Build history of the part. All positions in model axes, mm. A direction names the side the tool comes from. Round coordinates to 2 decimals unless told otherwise and drop trailing zeros. Write each loop counter-clockwise with the first axis right and the second up, starting at its lowest first coordinate (ties: lowest second). Pieces come first, ordered by that corner, then holes. Notation, with made-up numbers: M -6,35.25 L 28,35.25 A19 ccw 28,46.25 Z; hole C 12,80.5 d11. An arc over 180 degrees is marked long. Use a Markdown table: item, result.
from build123d import *

# Parameters (mm, degrees)
BOX001_W          = 5
BOX001_H          = 3
BOX001_DEPTH      = 10
BOX002_W          = 5
BOX002_H          = 3
BOX002_DEPTH      = 10
BOX003_W          = 5
BOX003_H          = 3
BOX003_DEPTH      = 10
CYLINDER_R        = 3.25
CYLINDER_DEPTH    = 10
CYLINDER002_R     = 1
CYLINDER002_DEPTH = 20
CYLINDER001_R     = 1
CYLINDER001_DEPTH = 20
CYLINDER004_R     = 1
CYLINDER004_DEPTH = 20
CYLINDER003_R     = 1
CYLINDER003_DEPTH = 20
CYLINDER006_R     = 1
CYLINDER006_DEPTH = 20
CYLINDER005_R     = 1
CYLINDER005_DEPTH = 20
CYLINDER008_R     = 1
CYLINDER008_DEPTH = 20
CYLINDER007_R     = 1
CYLINDER007_DEPTH = 20
BOX_W             = 29
BOX_H             = 8
BOX_DEPTH         = 11
FILLET_R          = 2


with BuildPart() as cube001:
    # Box001 → Box001 (new body)
    with BuildSketch(Plane(origin=(2, 1.5, 9), x_dir=(1, 0, 0), z_dir=(0, 0, 1))):
        with Locations((2.5, 1.5)):
            Rectangle(BOX001_W, BOX001_H)
    extrude(amount=BOX001_DEPTH)


with BuildPart() as cube002:
    # Box002 → Box002 (new body)
    with BuildSketch(Plane(origin=(8.35, 1.5, 9), x_dir=(1, 0, 0), z_dir=(0, 0, 1))):
        with Locations((2.5, 1.5)):
            Rectangle(BOX002_W, BOX002_H)
    extrude(amount=BOX002_DEPTH)


with BuildPart() as cube003:
    # Box003 → Box003 (new body)
    with BuildSketch(Plane(origin=(22.32, 1.5, 9), x_dir=(1, 0, 0), z_dir=(0, 0, 1))):
        with Locations((2.5, 1.5)):
            Rectangle(BOX003_W, BOX003_H)
    extrude(amount=BOX003_DEPTH)


with BuildPart() as cylinder:
    # Cylinder → Cylinder (new body)
    with BuildSketch(Plane(origin=(17, 3, 9), x_dir=(1, 0, 0), z_dir=(0, 0, 1))):
        Circle(CYLINDER_R)
    extrude(amount=CYLINDER_DEPTH)


with BuildPart() as cylinder002:
    # Cylinder002 → Cylinder002 (new body)
    with BuildSketch(Plane(origin=(5.75, 3, 0), x_dir=(1, 0, 0), z_dir=(0, 0, 1))):
        Circle(CYLINDER002_R)
    extrude(amount=CYLINDER002_DEPTH)


with BuildPart() as fusion:
    # Cylinder001 → Cylinder001 (new body)
    with BuildSketch(Plane(origin=(3.25, 3, 0), x_dir=(1, 0, 0), z_dir=(0, 0, 1))):
        Circle(CYLINDER001_R)
    extrude(amount=CYLINDER001_DEPTH)

    # Fusion: union Cylinder002
    add(cylinder002.part)


with BuildPart() as cylinder004:
    # Cylinder004 → Cylinder004 (new body)
    with BuildSketch(Plane(origin=(5.75, 3, 0), x_dir=(1, 0, 0), z_dir=(0, 0, 1))):
        Circle(CYLINDER004_R)
    extrude(amount=CYLINDER004_DEPTH)


with BuildPart() as fusion001:
    # Cylinder003 → Cylinder003 (new body)
    with BuildSketch(Plane(origin=(3.25, 3, 0), x_dir=(1, 0, 0), z_dir=(0, 0, 1))):
        Circle(CYLINDER003_R)
    extrude(amount=CYLINDER003_DEPTH)

    # Fusion001: union Cylinder004
    add(cylinder004.part)


with BuildPart() as fusion001_1:
    # Fusion001 placement: moved
    add(fusion001.part.moved(Location((6.25, 0, 0))))


with BuildPart() as cylinder006:
    # Cylinder006 → Cylinder006 (new body)
    with BuildSketch(Plane(origin=(5.75, 3, 0), x_dir=(1, 0, 0), z_dir=(0, 0, 1))):
        Circle(CYLINDER006_R)
    extrude(amount=CYLINDER006_DEPTH)


with BuildPart() as fusion002:
    # Cylinder005 → Cylinder005 (new body)
    with BuildSketch(Plane(origin=(3.25, 3, 0), x_dir=(1, 0, 0), z_dir=(0, 0, 1))):
        Circle(CYLINDER005_R)
    extrude(amount=CYLINDER005_DEPTH)

    # Fusion002: union Cylinder006
    add(cylinder006.part)


with BuildPart() as fusion002_1:
    # Fusion002 placement: moved
    add(fusion002.part.moved(Location((20.25, 0, 0))))


with BuildPart() as cylinder008:
    # Cylinder008 → Cylinder008 (new body)
    with BuildSketch(Plane(origin=(5.75, 3, 0), x_dir=(1, 0, 0), z_dir=(0, 0, 1))):
        Circle(CYLINDER008_R)
    extrude(amount=CYLINDER008_DEPTH)


with BuildPart() as fusion004:
    # Cylinder007 → Cylinder007 (new body)
    with BuildSketch(Plane(origin=(3.25, 3, 0), x_dir=(1, 0, 0), z_dir=(0, 0, 1))):
        Circle(CYLINDER007_R)
    extrude(amount=CYLINDER007_DEPTH)

    # Fusion003: union Cylinder008
    add(cylinder008.part)


with BuildPart() as fusion004_1:
    # Fusion003 placement: moved
    add(fusion004.part.moved(Location((12.5, 0, 0))))

    # Fusion004: union Cube001, Cube002, Cube003, Cylinder, Fusion, Fusion001, Fusion002
    add(cube001.part)
    add(cube002.part)
    add(cube003.part)
    add(cylinder.part)
    add(fusion.part)
    add(fusion001_1.part)
    add(fusion002_1.part)


with BuildPart() as standoff:
    # Box → Box (new body)
    with BuildSketch(Plane(origin=(0, -1, 0), x_dir=(1, 0, 0), z_dir=(0, 0, 1))):
        with Locations((14.5, 4)):
            Rectangle(BOX_W, BOX_H)
    extrude(amount=BOX_DEPTH)

    # Fillet
    fillet_edges = [standoff.edges().sort_by_distance(p)[0] for p in [
        (0, -1, 5.5),
        (0, 3, 11),
        (0, 7, 5.5),
        (29, -1, 5.5),
        (29, 3, 11),
        (29, 7, 5.5),
        (14.5, -1, 11),
        (14.5, 7, 11),
    ]]
    fillet(fillet_edges, radius=FILLET_R)

    # Cut: cut Fusion004
    add(fusion004_1.part, mode=Mode.SUBTRACT)


solid = standoff.part
Q1. Cut at B-B on x = 26. Give the cut face in (y, z).
Response values:
| item | result |
|---|---|
| outline | M -1,0 L 2,0 L 2,9 L 1.5,9 L 1.5,11 L 1,11 A2 ccw -1,9 Z; M 4,0 L 7,0 L 7,9 A2 ccw 5,11 L 4.5,11 L 4.5,9 L 4,9 Z |
Q2. Drop flat-ended pins along their axis: P1, Ø1.6, axis at x = 23.5, y = 3, coming from the -Z side (3 decimals); P2, Ø0.9, axis at x = 10, y = 2.5, coming from the +Z side; P3, Ø1.6, axis at x = 25.5, z = 10.5, coming from the -Y side; P4, Ø1.6, axis at y = 2.5, z = 10, coming from the -X side. Give the stop position or say it passes through.
Response values:
| item | result |
|---|---|
| P1 | passes through |
| P2 | stops at z = 9 |
| P3 | stops at y = -0.87 |
| P4 | stops at x = 0.01 |
Q3. Cut at D-D on y = 0.25. Give the cut face in (x, z).
Response values:
| item | result |
|---|---|
| outline | M 0.15,0 L 28.85,0 L 28.85,9 A1.85 ccw 27,10.85 L 18.73,10.85 L 18.73,9 L 15.27,9 L 15.27,10.85 L 2,10.85 A1.85 ccw 0.15,9 Z |
Q4. Drill centre lines: L1, parallel to Y at x = 9.5, z = 5; L2, parallel to Z at x = 18, y = 4.5; L3, parallel to X at y = 3, z = 9.85. Where is each one in solid material? Low to high.
Response values:
| item | result |
|---|---|
| L1 | y = -1 to 2, 4 to 7 |
| L2 | z = 0 to 9 |
| L3 | x = 0.19 to 2, 7 to 8.35, 13.35 to 13.75, 20.25 to 22.32, 27.32 to 28.81 |
Q5. Two-plate mould, pull along X, no slides. Class faces 3 (the flat face through (2, 3, 10)), 4 (the flat face through (22, 3, 11)), 5 (the cylindrical face through (0.57, 6.4, 4.56)): +X half, -X half, draft (parallel to the pull), parting line (faces both ways), or undercut.
Response values:
| item | result |
|---|---|
| face 3 | undercut |
| face 4 | draft |
| face 5 | -X half |
Q6. Cut at A-A on z = 8. Count the separate pieces of the cut face and the enclosed holes in it, and give its area (3 significant figures).
Response values:
| item | result |
|---|---|
| separate pieces | 1 |
| enclosed holes | 8 |
| area | 203 mm2 |
Q7. Which spindle directions (+Z, -Z, +X, -X, +Y, -Y) get a long thin tool onto all of the face, cutting with end or side? Do faces 1 (the flat face through (14, -1, 4)), 2 (the flat face through (13.35, 3, 10)). Say none if no direction does.
Response values:
| item | result |
|---|---|
| face 1 | +Z, -Z, +X, -X, -Y |
| face 2 | +Z |
Q8. Cut at C-C on x = 7.5. Give the cut face in (y, z).
Response values:
| item | result |
|---|---|
| outline | M -1,0 L 7,0 L 7,9 A2 ccw 5,11 L 1,11 A2 ccw -1,9 Z |
